Work out the finished part from the listing and answer in its coordinate system (mm). Face numbers are marked on the shaded views. A direction names the side the tool comes from. Round coordinates to 2 decimals unless told otherwise and drop trailing zeros. Write each loop counter-clockwise with the first axis right and the second up, starting at its lowest first coordinate (ties: lowest second). Pieces come first, ordered by that corner, then holes.
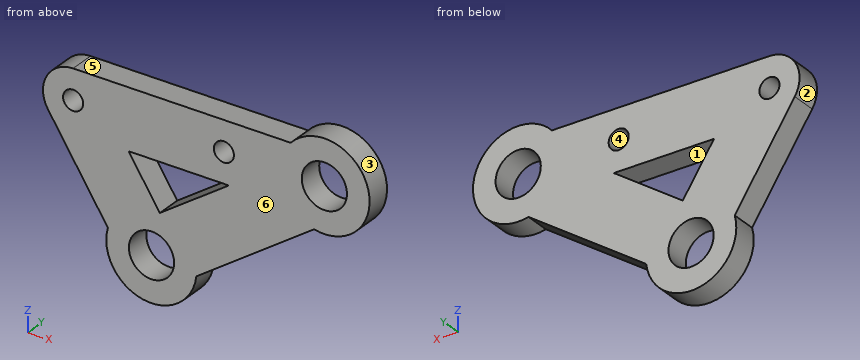
from build123d import *

# Parameters (mm, degrees)
SKETCH_1_R      = 2
SKETCH_1_R_2    = 4.5
EXTRUDE_1_DEPTH = 5


with BuildPart() as part:
    # 草图1 → 凸台-拉伸1 (new body)
    with BuildSketch(Plane(origin=(0, 0, 0), x_dir=(1, 0, 0), z_dir=(0, 1, 0))):
        with BuildLine():
            Line((-4.067495668, 16.82077086), (19.347989798, 0.425071426))
            ThreePointArc((19.347989798, 0.425071426), (29.985022701, -11.043860741), (14.693366212, -14.337508546))
            Line((14.693366212, -14.337508546), (-28.601114149, -14.337508546))
            ThreePointArc((-28.601114149, -14.337508546), (-33.872016823, -11.20414159), (-33.637695408, -5.076703549))
            Line((-33.637695408, -5.076703549), (-21.686265326, 13.383262263))
            ThreePointArc((-21.686265326, 13.383262263), (-14.727441536, 24.58696991), (-4.067495668, 16.82077086))
        make_face()
        with Locations(Location((1.398885851, -8.337508546, 0), (0, 0, 270))):
            Circle(SKETCH_1_R, mode=Mode.SUBTRACT)
        with Locations(Location((21.401570144, -8.337508546, 0), (0, 0, 270))):
            Circle(SKETCH_1_R_2, mode=Mode.SUBTRACT)
        with Locations(Location((-28.601114149, -8.337508546, 0), (0, 0, 270))):
            Circle(SKETCH_1_R, mode=Mode.SUBTRACT)
        with Locations(Location((-13.003993251, 15.7535263, 0), (0, 0, 270))):
            Circle(SKETCH_1_R_2, mode=Mode.SUBTRACT)
        Polygon((-11.348795412, 7.269896763), (2.37200133, -2.337508546), (-17.56886288, -2.337508546), align=None, mode=Mode.SUBTRACT)
    extrude(amount=EXTRUDE_1_DEPTH)


solid = part.part
Q1. Find the intervals of material crossed by L1, parallel to Z at x = -16.5, y = 2.7; L2, parallel to Z at x = 18, y = 3.65; L3, parallel to Z at x = -14, y = 3.05, in increasing order.
Q2. Find section B-B (x = 24.5). Determine the outline of the cut face in (y, z).
Q3. Find section C-C (y = 1.8). Determine the outline of the cut face in (x, z).
Q4. Find section D-D (x = -15). Determine the outline of the cut face in (y, z), plus the area to 3 significant figures.
Q5. The mould has two halves that part along Z. Classify the marked faces 3, 4, 5 and 6: +Z half, -Z half, draft (parallel to the pull), parting line (faces both ways), or undercut.
Q6. Find section A-A (z = 11). Determine the outline of the cut face in (x, y).
Q7. Given pin 1 (1 mm diameter, centred on x = 17.5, y = 4, fed in from -Z); pin 2 (2.5 mm diameter, centred on x = -9.5, y = 2.5, fed in from -Z); pin 3 (6.5 mm diameter, centred on x = -28.6, z = 8.34, fed in from +Y); pin 4 (1 mm diameter, centred on y = 1, z = -14, fed in from +X), each flat-ended and moving along its own axis, determine where each tip first touches the part or whether it passes through.
Q8. A tool of negligible diameter and unlimited length cuts with its end or side. For the marked faces 1 and 2, from which of +Z, -Z, +X, -X, +Y, -Y can it reach the whole face along a straight path? Write none if from no direction.
Report:
1. L1: z = -24.05 to -18.59, -12.92 to 0.69, 2.34 to 14.34
1. L2: z = -1.37 to 5.39, 11.28 to 16.67
1. L3: z = -24.7 to -20.14, -11.37 to -3.17, 2.34 to 14.34
2. outline: (0, -0.11) - (5, -0.11) - (5, 5.07) - (0, 5.07) - close; (0, 11.6) - (5, 11.6) - (5, 16.79) - (0, 16.79) - close
3. outline: (-33.64, 5.08) - (-21.69, -13.38) arc R9 ccw (long way) to (-4.07, -16.82) - (19.35, -0.43) arc R9 ccw (long way) to (14.69, 14.34) - (-28.6, 14.34) arc R6 ccw to start; hole circle Ø4 at (-28.6, 8.34); hole (-17.57, 2.34) - (-11.35, -7.27) - (2.37, 2.34) - close; hole circle Ø9 at (-13, -15.75); hole circle Ø4 at (1.4, 8.34); hole circle Ø9 at (21.4, 8.34)
4. outline: (0, -24.53) - (5, -24.53) - (5, -19.79) - (0, -19.79) - close; (0, -11.72) - (5, -11.72) - (5, -1.63) - (0, -1.63) - close; (0, 2.34) - (5, 2.34) - (5, 14.34) - (0, 14.34) - close
4. area: 134 mm2
5. face 3: parting line
5. face 4: undercut
5. face 5: +Z half
5. face 6: draft
6. outline: (-33.98, 0) - (17.77, 0) - (17.77, 5) - (-33.98, 5) - close; (25.03, 0) - (30, 0) - (30, 5) - (25.03, 5) - close
7. pin 1: stops at z = -2.07
7. pin 2: stops at z = -24.47
7. pin 3: stops at y = 5
7. pin 4: stops at x = 0.68
8. face 1: +Y, -Y
8. face 2: -X, +Y, -Y
